from build123d import *

# Parameters (mm, degrees)
BOSS_EXTRUDE1_DEPTH = 125


with BuildPart() as part:
    # Sketch1 → Boss-Extrude1 (new, symmetric)
    with BuildSketch(Plane(origin=(0, 0, 0), x_dir=(0, 0, -1), z_dir=(1, 0, 0))):
        with BuildLine():
            Line((-15, 10), (15, 10))
            ThreePointArc((15, 10), (18.535533906, 8.535533906), (20, 5))
            Line((20, 5), (20, -5))
            ThreePointArc((20, -5), (18.535533906, -8.535533906), (15, -10))
            Line((15, -10), (-15, -10))
            ThreePointArc((-15, -10), (-18.535533906, -8.535533906), (-20, -5))
            Line((-20, -5), (-20, 5))
            ThreePointArc((-20, 5), (-18.535533906, 8.535533906), (-15, 10))
        make_face()
        with BuildLine():
            Line((-8.870332019, 5), (8.870332019, 5))
            ThreePointArc((8.870332019, 5), (12.784941828, 3.587180501), (14.895004608, 0))
            ThreePointArc((14.895004608, 0), (12.784941828, -3.587180501), (8.870332019, -5))
            Line((8.870332019, -5), (-8.870332019, -5))
            ThreePointArc((-8.870332019, -5), (-12.784941828, -3.587180501), (-14.895004608, 0))
            ThreePointArc((-14.895004608, 0), (-12.784941828, 3.587180501), (-8.870332019, 5))
        make_face(mode=Mode.SUBTRACT)
    extrude(amount=BOSS_EXTRUDE1_DEPTH, both=True)


solid = part.part
Can you work these out from the model? Positions are in its coordinate system, mm. A direction names the side the tool comes from. Give positions to 0.01 mm unless a question says otherwise; leave off trailing zeros. Loops run counter-clockwise (first coordinate to the right, second up) from the corner with the lowest first, then second, coordinate; pieces in that order, holes last. Notation, with made-up numbers: (37.25, -12) -> (49.25, -12) arc R25 ccw to (49.25, 23) -> close; hole circle Ø2 at (7.5, 89). An arc over 180 degrees is marked (long way). Use one line per item in the form item = value.
1) I need wall thicknesses on line 1 along Y through (x, z) = (12.5, 2); line 2 along Z through (x, y) = (43, 3.25); line 3 along Z through (x, y) = (63.5, 4). Which ranges of each line are inside material? Lowest first, please.
Answers:
line_1 = -10 to -5, 5 to 10
line_2 = -20 to -13.16, 13.16 to 20
line_3 = -20 to -12.23, 12.23 to 20
2) Will this pin go through, and if not, where does the flat tip stop? pin 1 (2 mm diameter, centred on y = -3, z = -0.5, fed in from +X).
Answers:
pin_1 = through
3) For faces 4 (the face through (2, 9, -18)), 5 (the face through (1.75, 3.625, -12.739)), which set-ups out of +Z, -Z, +X, -X, +Y, -Y let a thin tool reach every point of the face, with its end or its side?
Answers:
face_4 = -Z, +X, -X, +Y
face_5 = +X, -X
4) If we section it at B-B (x = -88): Please give me the cut outline in (y, z) (3 decimals).
Answers:
outline = (-10, -15) arc R5 ccw to (-5, -20) -> (5, -20) arc R5 ccw to (10, -15) -> (10, 15) arc R5 ccw to (5, 20) -> (-5, 20) arc R5 ccw to (-10, 15) -> close; hole (-5, -8.87) arc R6.13 ccw to (0, -14.895) arc R6.13 ccw to (5, -8.87) -> (5, 8.87) arc R6.13 ccw to (0, 14.895) arc R6.13 ccw to (-5, 8.87) -> close
5) We'd pull the mould along Z, two halves only. Please class faces 1 (the face through (2, -9, 18)), 2 (the face through (125, -7, 0)), 3 (the face through (1.75, -3.625, 12.739)): released by +Z, released by -Z, zero draft, split by the parting line, or undercut.
Answers:
face_1 = released by +Z
face_2 = zero draft
face_3 = undercut
6) If we section it at A-A (z = 3): Please give me the cut outline in (x, y), plus the area to 3 significant figures.
Answers:
outline = (-125, -10) -> (125, -10) -> (125, -5) -> (-125, -5) -> close; (-125, 5) -> (125, 5) -> (125, 10) -> (-125, 10) -> close
area = 2,500 mm²
7) If we section it at C-C (y = 7.5): Please give me the cut outline in (x, z).
Answers:
outline = (-125, -19.33) -> (125, -19.33) -> (125, 19.33) -> (-125, 19.33) -> close
